Model file for the job. Use its own axes, mm. A direction names the side the tool comes from. Give positions to 0.01 mm unless a question says otherwise; leave off trailing zeros. Write each loop counter-clockwise with the first axis right and the second up, starting at its lowest first coordinate (ties: lowest second). Pieces come first, ordered by that corner, then holes. Notation, with made-up numbers: (14, 33) - (49, 33) arc R14 cw to (49, 53) - close; hole circle Ø2 at (2, 22). An arc over 180 degrees is marked (long way). Use a Markdown table: item, result. Add a question column.
Autodesk Inventor part; units mm, degrees
ref_plane "Work Plane1" through (0, 22, 0) normal (0, 1, 0) x (-1, 0, 0)
ref_plane "Work Plane2" through (-25, 0, 0) normal (1, 0, 0) x (0, 1, 0)
ref_plane "XY Plane" through (0, 0, 0) normal (0, 0, 1) x (1, 0, 0)
sketch "Sketch1" plane through (0, 0, 0) normal (1, 0, 0) x (0, 1, 0)
  line L0 (11, 10) -> (11, 4)
  line L1 (11, 4) -> (16, 4)
  line L2 (16, 4) -> (16, -4)
  line L3 (16, -4) -> (-16, -4)
  line L4 (-16, -4) -> (-16, 4)
  line L5 (-16, 4) -> (-11, 4)
  line L6 (-11, 4) -> (-11, 10)
  line L7 (-11, 10) -> (-22, 10)
  line L8 (-22, 10) -> (-22, -10)
  line L9 (-22, -10) -> (22, -10)
  line L10 (22, -10) -> (22, 10)
  line L11 (22, 10) -> (11, 10)
  line L12 (11, 7) -> (-11, 7) construction
  line L13 (16, 0) -> (-16, 0) construction
  point P0 (0, 0)
  point P1 (-13.5, 4)
  point P2 (13.5, 4)
  point P3 (16.5, 10)
  point P4 (-16.5, 10)
  point P5 (22, 0)
  point P6 (0, -10)
  point P7 (0, 7)
  point P8 (0, 0)
  dimension "d0" = 22
  dimension "d1" = 32
  dimension "d2" = 6
  dimension "d3" = 14
  dimension "d4" = 44
  dimension "d5" = 20
extrude "Extrusion1" add sketch "Sketch1" along normal mid plane 50
ref_plane "Work Plane1" through (0, 22, 0) normal (0, 1, 0) x (-1, 0, 0)
sketch "Sketch2" plane through (0, 22, 0) normal (0, 1, 0) x (-1, 0, 0)
  line L0 (25, 10) -> (-25, 10) construction
  line L1 (-25, -10) -> (-25, 10) construction
  line L2 (25, -10) -> (-25, -10) construction
  line L3 (25, 10) -> (25, -10) construction
  line L4 (-25, 0) -> (25, 0) construction
  circle A0 centre (0, 0) radius 2.75
  point P0 (0, 0)
  dimension "d9" = 5.5
  dimension "d10" = 25
extrude "Extrusion2" cut sketch "Sketch2" against normal up to surface (6 mm away)
sketch "Sketch3" plane through (0, 22, 0) normal (0, 1, 0) x (-1, 0, 0)
  line L0 (22, 4) -> (19.2, 4)
  line L1 (19.2, 4) -> (19.2, -4)
  line L2 (19.2, -4) -> (22, -4)
  line L3 (22, -4) -> (22, 4)
  line L4 (25, 10) -> (25, -10) construction
  point P0 (0, 0)
  point P1 (19.2, 0)
  dimension "d13" = 8
  dimension "d14" = 3
  dimension "d15" = 2.8
extrude "Extrusion3" cut sketch "Sketch3" against normal through all
ref_plane "Work Plane2" through (-25, 0, 0) normal (1, 0, 0) x (0, 1, 0)
sketch "Sketch4" plane through (-25, 0, 0) normal (1, 0, 0) x (0, 1, 0)
  circle A0 centre (19, 0) radius 2.75
  line L0 (0, -10) -> (0, 10) construction
  line L1 (22, -10) -> (-22, -10) construction
  circle A1 centre (-19, 0) radius 2.75
  point P0 (0, 0)
  point P1 (11, 10)
  point P2 (0, 0)
  dimension "d19" = 5.5
  dimension "d20" = 19
extrude "Extrusion4" cut sketch "Sketch4" along normal blind 10
properties part number "cuerpo_obj2"
(1) Band-saw the part on D-D (x = -6.5). Write the cut outline in (y, z).
(2) Probe probe 1 along Y at (x, z) = (-4.5, -1.75); probe 2 along Y at (x, z) = (-17.15, 0); probe 3 along Z at (x, y) = (-23, 19). List the from-to ranges inside material, lowest first. Write a range as [from, to].
(3) Flat gauge pins, fed straight in: pin 1 (2 mm diameter, centred on x = -1, y = 1, fed in from +Z); pin 2 (1.6 mm diameter, centred on y = 18, z = -1, fed in from -X). Where does each tip first touch, or does it go through?
(4) Which spindle directions (+Z, -Z, +X, -X, +Y, -Y) get a long thin tool onto all of the face, cutting with end or side? Do faces 1 (the cylindrical face through (-17.129, 16.253, -0.121)), 2 (the cylindrical face through (0.596, 19.042, -2.685)), 3 (the flat face through (0, -11, 7)). Say none if no direction does.
(5) Band-saw the part on A-A (y = 12). Write the cut outline in (x, z), then the cut area to 3 significant figures.
(6) Band-saw the part on B-B (x = 0). Write the cut outline in (y, z).
(7) Two-plate mould, pull along Y, no slides. Class faces 4 (the flat face through (0, 22, 4)), 5 (the flat face through (-19.2, 18, 3)), 6 (the flat face through (-24, 16, 0)): +Y half, -Y half, draft (parallel to the pull), parting line (faces both ways), or undercut.
(8) Band-saw the part on C-C (z = 6.75). Write the cut outline in (x, y).
Model answer:
| question | item | result |
|---|---|---|
| 1 | outline | (-22, -10) - (22, -10) - (22, 10) - (11, 10) - (11, 4) - (16, 4) - (16, -4) - (-16, -4) - (-16, 4) - (-11, 4) - (-11, 10) - (-22, 10) - close |
| 2 | probe 1 | y = [-22, -16], [16, 22] |
| 2 | probe 2 | y = [-22, -21.75], [-16.25, -16], [16, 16.25], [21.75, 22] |
| 2 | probe 3 | z = [-10, -2.75], [2.75, 10] |
| 3 | pin 1 | stops at z = -4 |
| 3 | pin 2 | stops at x = -15 |
| 4 | face 1 | -X |
| 4 | face 2 | +Y |
| 4 | face 3 | +Z, +X, -X |
| 5 | outline | (-25, -10) - (25, -10) - (25, -4) - (-25, -4) - close; (-25, 4) - (25, 4) - (25, 10) - (-25, 10) - close |
| 5 | area | 600 mm^2 |
| 6 | outline | (-22, -10) - (22, -10) - (22, -2.75) - (16, -2.75) - (16, -4) - (-16, -4) - (-16, 4) - (-11, 4) - (-11, 10) - (-22, 10) - close; (11, 4) - (16, 4) - (16, 2.75) - (22, 2.75) - (22, 10) - (11, 10) - close |
| 7 | face 4 | +Y half |
| 7 | face 5 | draft |
| 7 | face 6 | undercut |
| 8 | outline | (-25, -22) - (25, -22) - (25, -11) - (-25, -11) - close; (-25, 11) - (25, 11) - (25, 22) - (-25, 22) - close |
